from build123d import *

# Parameters (mm, degrees)
SKETCH_R  = 2.1
PAD_DEPTH = 1


with BuildPart() as part:
    # Sketch → Pad (new body)
    with BuildSketch(Plane.XY):
        with BuildLine():
            Line((5, 15), (23.5, 15))
            ThreePointArc((25, 13.5), (24.56066, 14.56066), (23.5, 15))
            Line((25, 13.5), (25, -3.5))
            ThreePointArc((23.5, -5), (24.56066, -4.56066), (25, -3.5))
            Line((23.5, -5), (-3.5, -5))
            ThreePointArc((-5, -3.5), (-4.56066, -4.56066), (-3.5, -5))
            Line((-5, -3.5), (-5, 5))
            ThreePointArc((-4.56066, 6.06066), (-4.885819, 5.574025), (-5, 5))
            Line((-4.56066, 6.06066), (3.93934, 14.56066))
            ThreePointArc((5, 15), (4.425975, 14.885819), (3.93934, 14.56066))
        make_face()
        Circle(SKETCH_R, mode=Mode.SUBTRACT)
        with Locations((10, 0)):
            Circle(SKETCH_R, mode=Mode.SUBTRACT)
        with Locations((20, 0)):
            Circle(SKETCH_R, mode=Mode.SUBTRACT)
        with Locations((10, 10)):
            Circle(SKETCH_R, mode=Mode.SUBTRACT)
        with Locations((20, 10)):
            Circle(SKETCH_R, mode=Mode.SUBTRACT)
    extrude(amount=PAD_DEPTH)


solid = part.part
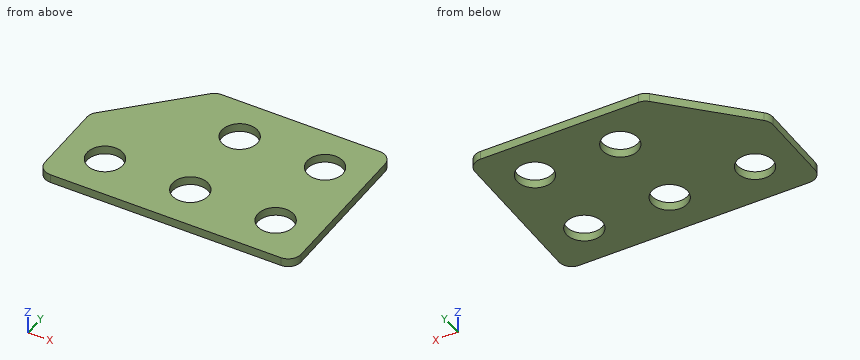
Geometry: final body of the model. Coordinates: model frame, mm. Give positions to 0.01 mm unless a question says otherwise; leave off trailing zeros. Write each loop counter-clockwise with the first axis right and the second up, starting at its lowest first coordinate (ties: lowest second). Pieces come first, ordered by that corner, then holes. Notation, with made-up numbers: M 1,-25 L 57,-25 A29 cw 57,2 Z; hole C 30,83.25 d8. An arc over 180 degrees is marked long. Answer in a Markdown table with one row per item. Add a question column.
(1) Section D-D on x = 0. Return loops of the section in (y, z), and give its area (3 significant figures).
(2) Section C-C on y = 0. Return loops of the section in (x, z).
(3) Ray query, line 1 (Y direction, x = 20, z = 0.7); line 2 (Y direction, x = 20.5, z = 0.85); line 3 (X direction, y = 9.25, z = 0.7). Return the intervals inside material, ascending.
(4) Section B-B on z = 0.85. Return loops of the section in (x, y), and give its area (3 significant figures).
(5) Section A-A on x = 10. Return loops of the section in (y, z).
Result set:
| question | item | result |
|---|---|---|
| 1 | outline | M -5,0 L -2.1,0 L -2.1,1 L -5,1 Z; M 2.1,0 L 10.62,0 L 10.62,1 L 2.1,1 Z |
| 1 | area | 11.4 mm^2 |
| 2 | outline | M -5,0 L -2.1,0 L -2.1,1 L -5,1 Z; M 2.1,0 L 7.9,0 L 7.9,1 L 2.1,1 Z; M 12.1,0 L 17.9,0 L 17.9,1 L 12.1,1 Z; M 22.1,0 L 25,0 L 25,1 L 22.1,1 Z |
| 3 | line 1 | y = -5 to -2.1, 2.1 to 7.9, 12.1 to 15 |
| 3 | line 2 | y = -5 to -2.04, 2.04 to 7.96, 12.04 to 15 |
| 3 | line 3 | x = -1.37 to 8.04, 11.96 to 18.04, 21.96 to 25 |
| 4 | outline | M -5,-3.5 A1.5 ccw -3.5,-5 L 23.5,-5 A1.5 ccw 25,-3.5 L 25,13.5 A1.5 ccw 23.5,15 L 5,15 A1.5 ccw 3.94,14.56 L -4.56,6.06 A1.5 ccw -5,5 Z; hole C 0,0 d4.2; hole C 10,0 d4.2; hole C 10,10 d4.2; hole C 20,0 d4.2; hole C 20,10 d4.2 |
| 4 | area | 485 mm^2 |
| 5 | outline | M -5,0 L -2.1,0 L -2.1,1 L -5,1 Z; M 2.1,0 L 7.9,0 L 7.9,1 L 2.1,1 Z; M 12.1,0 L 15,0 L 15,1 L 12.1,1 Z |
